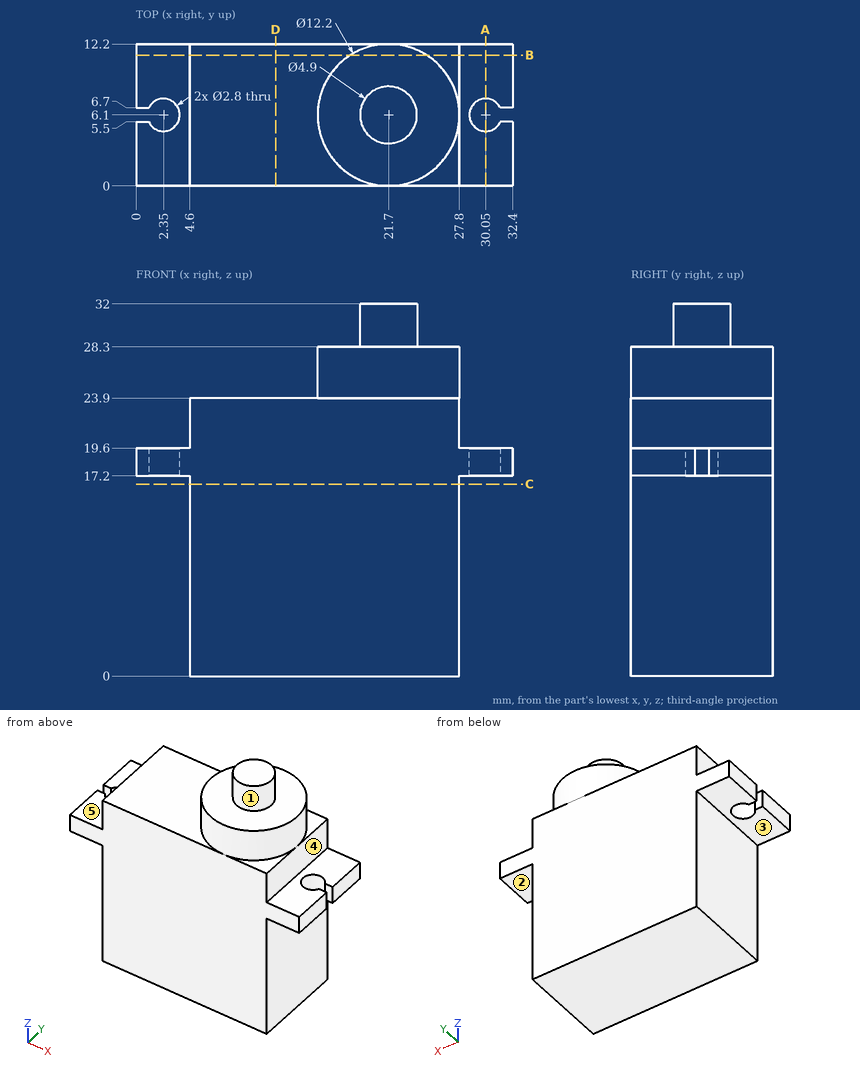
Could you check a few things on this drawing? It's one solid part, dimensions in mm from its lowest x, y, z. A direction names the side the tool comes from. Give positions to 0.01 mm unless a question says otherwise; leave off trailing zeros. Loops run counter-clockwise (first coordinate to the right, second up) from the corner with the lowest first, then second, coordinate; pieces in that order, holes last. Notation, with made-up numbers: M 58,31 L 95,31 A23 cw 95,51 Z; hole C 10,68 d5. An arc over 180 degrees is marked long. Answer as a JSON object with one key per item and string values.
Q1. Suppose I cut it at A-A, the plane x = 30.05. List the corners of the cut face in (y, z) for me.
Values found:
{"outline": "M 0,17.2 L 4.7,17.2 L 4.7,19.6 L 0,19.6 Z; M 7.5,17.2 L 12.2,17.2 L 12.2,19.6 L 7.5,19.6 Z"}
Q2. Suppose I cut it at B-B, the plane y = 11.25. List the corners of the cut face in (x, z) for me.
Values found:
{"outline": "M 0,17.2 L 4.6,17.2 L 4.6,0 L 27.8,0 L 27.8,17.2 L 32.4,17.2 L 32.4,19.6 L 27.8,19.6 L 27.8,23.9 L 24.97,23.9 L 24.97,28.3 L 18.43,28.3 L 18.43,23.9 L 4.6,23.9 L 4.6,19.6 L 0,19.6 Z"}
Q3. Suppose I cut it at D-D, the plane x = 12. List the corners of the cut face in (y, z) for me.
Values found:
{"outline": "M 0,0 L 12.2,0 L 12.2,23.9 L 0,23.9 Z"}
Q4. For the marked faces 1, 2, 3, 4 and 5, which set-ups out of +Z, -Z, +X, -X, +Y, -Y let a thin tool reach every point of the face, with its end or its side?
Values found:
{"face 1": "+Z", "face 2": "-Z, +X, +Y, -Y", "face 3": "-Z, -X, +Y, -Y", "face 4": "+Z, +X, +Y, -Y", "face 5": "+Z, -X, +Y, -Y"}
Q5. Suppose I cut it at C-C, the plane z = 16.5. List the corners of the cut face in (x, y) for me.
Values found:
{"outline": "M 4.6,0 L 27.8,0 L 27.8,12.2 L 4.6,12.2 Z"}
Q6. If I drill on probe 1 along Y at (x, z) = (2.35, 18.8); probe 2 along Z at (x, y) = (12, 9.5); probe 3 along X at (y, z) = (9.5, 20.5), over which ranges is the centre line in solid material (lowest first)? Write a range as [from, to].
Values found:
{"probe 1": "y = [0, 4.7], [7.5, 12.2]", "probe 2": "z = [0, 23.9]", "probe 3": "x = [4.6, 27.8]"}
Q7. For P1, Ø5, axis at x = 24.5, y = 4.5, coming from the +Z side; P2, Ø1, axis at y = 8, z = 21, coming from the -X side; P3, Ø3.5, axis at x = 30.5, y = 7.5, coming from the +Z side; P4, Ø6, axis at y = 1.5, z = 12.5, coming from the +X side, each with a flat end and sliding along its axis, tell me the tip position at first contact or that it passes through.
Values found:
{"P1": "stops at z = 32", "P2": "stops at x = 4.6", "P3": "stops at z = 19.6", "P4": "stops at x = 27.8"}
